Check sheet for the modelled part. Datum: model origin and axes. Units: mm. Face numbers are marked on the shaded views. Coordinates: 2 decimals unless noted, no trailing zeros. Loops run counter-clockwise (first coordinate to the right, second up) from the corner with the lowest first, then second, coordinate; pieces in that order, holes last.
```python
from build123d import *

# Parameters (mm, degrees)
SKETCH1_W           = 149.352
SKETCH1_H           = 66.04
BOSS_EXTRUDE1_DEPTH = 23.3045
FILLET1_R           = 9.525
CUT_EXTRUDE1_DEPTH  = 25.4


with BuildPart() as part:
    # Sketch1 → Boss-Extrude1 (new, symmetric)
    with BuildSketch(Plane(origin=(0, 0, 0), x_dir=(1, 0, 0), z_dir=(0, 1, 0))):
        Rectangle(SKETCH1_W, SKETCH1_H)
    extrude(amount=BOSS_EXTRUDE1_DEPTH, both=True)

    # Fillet1
    fillet1_edges = [part.edges().sort_by_distance(p)[0] for p in [
        (74.676, 23.3045, 0),
        (-74.676, 23.3045, 0),
        (74.676, -23.3045, 0),
        (-74.676, -23.3045, 0),
    ]]
    fillet(fillet1_edges, radius=FILLET1_R)

    # Sketch2 → Cut-Extrude1 (cut, symmetric)
    with BuildSketch(Plane.XY):
        with BuildLine():
            Line((-74.676, 10.16), (-74.676, -10.16))
            ThreePointArc((-74.676, -10.16), (-71.700204897, -2.975795103), (-64.516, 0))
            ThreePointArc((-64.516, 0), (-71.700204897, 2.975795103), (-74.676, 10.16))
        make_face()
    cut_extrude1 = extrude(amount=CUT_EXTRUDE1_DEPTH, both=True, mode=Mode.SUBTRACT)

    # Mirror1: Cut-Extrude1 across plane
    add(cut_extrude1.mirror(Plane(origin=(0, 0, 0), x_dir=(0, 0, 1), z_dir=(1, 0, 0))), mode=Mode.SUBTRACT)


solid = part.part
```
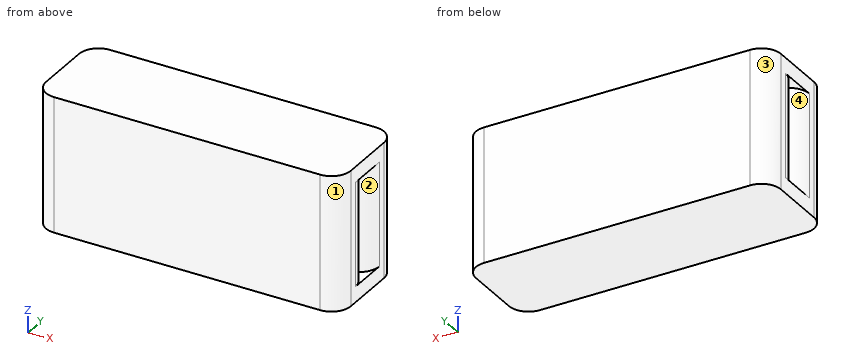
1) Scan lines: line 1 (X direction, y = 9.5, z = -20.5); line 2 (X direction, y = 16, z = -2). Record each from-to range of solid material in increasing order.
Answer sheet:
line 1: x = -74.65 to 74.65
line 2: x = -74.41 to 74.41
2) Section check B-B on y = -18.5. Enter the section's corners in (x, z).
Answer sheet:
outline: (-73.42, -33.02) - (73.42, -33.02) - (73.42, 33.02) - (-73.42, 33.02) - close
3) Depth check by flat-ended pin: pin 1 (5 mm diameter, centred on y = 8.5, z = -14.5, fed in from -X). Enter the tip coordinate at first touch or a pass-through.
Answer sheet:
pin 1: stops at x = -74.68
4) Mould release check, pull along Y, two halves, no side actions. Record for the marked faces 1, 2, 3 and 4: +Y half, -Y half, draft (parallel to the pull), parting line (faces both ways), or undercut.
Answer sheet:
face 1: -Y half
face 2: undercut
face 3: +Y half
face 4: undercut
